```python
from build123d import *

# Parameters (mm, degrees)
SKETCH1_W           = 609.6
SKETCH1_H           = 304.8
BOSS_EXTRUDE1_DEPTH = 254
SHELL1_T            = -12.7
SKETCH2_W           = 24.13
SKETCH2_H           = 276.86
BOSS_EXTRUDE3_DEPTH = 241.3


with BuildPart() as part:
    # Sketch1 → Boss-Extrude1 (new body)
    with BuildSketch(Plane(origin=(0, 0, 0), x_dir=(1, 0, 0), z_dir=(0, 1, 0))):
        Rectangle(SKETCH1_W, SKETCH1_H)
    extrude(amount=BOSS_EXTRUDE1_DEPTH)

    # Shell1
    shell1_openings = [part.faces().sort_by_distance(p)[0] for p in [
        (0, 254, 0),
    ]]
    offset(amount=SHELL1_T, openings=shell1_openings, kind=Kind.INTERSECTION)

    # Sketch2 → Boss-Extrude3 (add)
    with BuildSketch(Plane(origin=(0, 12.7, 0), x_dir=(1, 0, 0), z_dir=(0, 1, 0))):
        with Locations((-278.765, 0)):
            Rectangle(SKETCH2_W, SKETCH2_H)
    boss_extrude3 = extrude(amount=BOSS_EXTRUDE3_DEPTH)

    # Mirror1: Boss-Extrude3 across plane
    add(boss_extrude3.mirror(Plane(origin=(0, 0, 0), x_dir=(0, 0, 1), z_dir=(1, 0, 0))))


solid = part.part
```
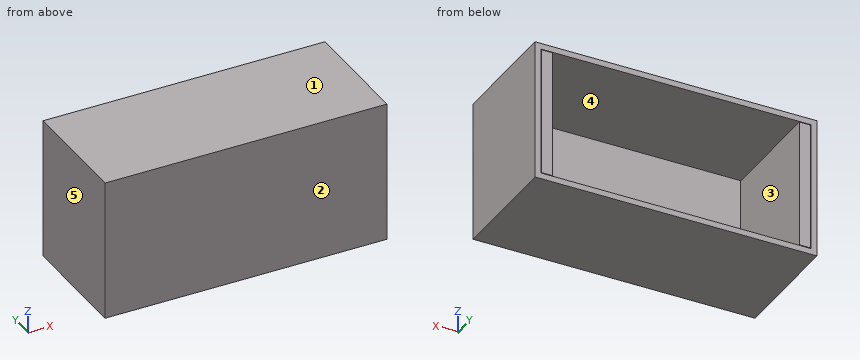
Geometry check sheet. Reference: the model listing, model coordinates, mm. Face numbers are marked on the shaded views. A direction names the side the tool comes from. Give positions to 0.01 mm unless a question says otherwise; leave off trailing zeros. Order: outer loops, then holes, each group sorted by start corner. A loop starts at its lowest first (then second) coordinate and runs counter-clockwise, first axis right, second up.
1. Section check C-C, the plane x = 101. Enter the section's corners in (y, z), and give its area (4 significant figures).
2. Section check A-A, the plane y = 205. Enter the section's corners in (x, z), and give its area (3 significant figures).
3. Release check for a two-part mould opening along Z. For the marked faces 1, 2 and 3 record: pulls with the +Z half, pulls with the -Z half, needs draft (parallel to the pull), parting line crosses it, or undercut.
4. Section check B-B, the plane z = -51. Enter the section's corners in (x, y).
5. Gauge pin test, flat end, axial feed: pin 1 Ø1.5 at (x, z) = (-194.5, 57) entering from +Y. Record the tip position at first contact, or that the pin passes through.
6. Thickness scan on L1, parallel to X at y = 75.5, z = 125; L2, parallel to Z at x = 101.5, y = 17; L3, parallel to X at y = 71, z = 138.5. Record the ranges inside material, lowest first.
7. Access from +Z, -Z, +X, -X, +Y, -Y to the whole of each face (thin tool, end or side, straight path). Record for the marked faces 4 and 5.
Values follow:
1. outline: (0, -152.4) - (254, -152.4) - (254, -139.7) - (12.7, -139.7) - (12.7, 139.7) - (254, 139.7) - (254, 152.4) - (0, 152.4) - close
1. area: 10,000 mm2
2. outline: (-304.8, -152.4) - (304.8, -152.4) - (304.8, 152.4) - (-304.8, 152.4) - close; (-290.83, -138.43) - (-266.7, -138.43) - (-266.7, 138.43) - (-290.83, 138.43) - close; (266.7, -138.43) - (290.83, -138.43) - (290.83, 138.43) - (266.7, 138.43) - close; hole (-292.1, -139.7) - (292.1, -139.7) - (292.1, 139.7) - (-292.1, 139.7) - close
2. area: 35,900 mm2
3. face 1: pulls with the +Z half
3. face 2: needs draft
3. face 3: undercut
4. outline: (-304.8, 0) - (304.8, 0) - (304.8, 254) - (292.1, 254) - (292.1, 12.7) - (290.83, 12.7) - (290.83, 254) - (266.7, 254) - (266.7, 12.7) - (-266.7, 12.7) - (-266.7, 254) - (-290.83, 254) - (-290.83, 12.7) - (-292.1, 12.7) - (-292.1, 254) - (-304.8, 254) - close
5. pin 1: stops at y = 12.7
6. L1: x = -304.8 to -292.1, -290.83 to -266.7, 266.7 to 290.83, 292.1 to 304.8
6. L2: z = -152.4 to -139.7, 139.7 to 152.4
6. L3: x = -304.8 to -292.1, 292.1 to 304.8
7. face 4: +Y
7. face 5: +Z, -Z, -X, +Y, -Y
